Read the model definition and answer for the solid it produces. Units are mm, in the model's axes. A direction names the side the tool comes from. Coordinates: 2 decimals unless noted, no trailing zeros. Order: outer loops, then holes, each group sorted by start corner. A loop starts at its lowest first (then second) coordinate and runs counter-clockwise, first axis right, second up.
```python
from build123d import *

# Parameters (mm, degrees)
SKETCH1_R                = 10.975
SKETCH1_R_2              = 1.7
BOSS_EXTRUDE1_DEPTH      = 3.6
SKETCH2_R                = 5.125
BOSS_EXTRUDE2_DEPTH      = 13.7
BOSS_EXTRUDE3_DEPTH      = 13.7
BOSS_EXTRUDE3_DEPTH_BACK = 1.3
SKETCH2_2_R              = 5.125
CUT_EXTRUDE1_DEPTH       = 21.702445508
CUT_EXTRUDE1_DEPTH_BACK  = 21.702445508
SKETCH3_R                = 3.325
FILLET1_R                = 0.2
CHAMFER1_SIZE            = 0.2


with BuildPart() as part:
    # Sketch1 → Boss-Extrude1 (new body)
    with BuildSketch(Plane(origin=(0, 0, 0), x_dir=(0, 0, -1), z_dir=(1, 0, 0))):
        Circle(SKETCH1_R)
        with Locations((0, 7.775)):
            Circle(SKETCH1_R_2, mode=Mode.SUBTRACT)
        with Locations((7.775, 0)):
            Circle(SKETCH1_R_2, mode=Mode.SUBTRACT)
        with Locations((0, -7.775)):
            Circle(SKETCH1_R_2, mode=Mode.SUBTRACT)
        with Locations((-7.775, 0)):
            Circle(SKETCH1_R_2, mode=Mode.SUBTRACT)
    extrude(amount=BOSS_EXTRUDE1_DEPTH)

    # Sketch2 → Boss-Extrude2 (add)
    with BuildSketch(Plane(origin=(0, 0, 0), x_dir=(0, 0, -1), z_dir=(1, 0, 0))):
        with Locations(Location((0, 0, 0), (0, 0, 180))):
            Circle(SKETCH2_R)
    extrude(amount=BOSS_EXTRUDE2_DEPTH)

    # Sketch2_2 → Boss-Extrude3 (add, two sides: drawn at the far end of the back side and taken through both)
    with BuildSketch(Plane(origin=(0, 0, 0), x_dir=(0, 0, -1), z_dir=(1, 0, 0)).offset(-BOSS_EXTRUDE3_DEPTH_BACK)):
        with Locations(Location((0, 0, 0), (0, 0, 180))):
            Circle(SKETCH2_2_R)
    extrude(amount=BOSS_EXTRUDE3_DEPTH + BOSS_EXTRUDE3_DEPTH_BACK)

    # Sketch3 → Cut-Extrude1 (cut, two sides: drawn at the far end of the back side and taken through both)
    with BuildSketch(Plane(origin=(0, 0, 0), x_dir=(0, 0, -1), z_dir=(1, 0, 0)).offset(-CUT_EXTRUDE1_DEPTH_BACK)):
        Circle(SKETCH3_R)
    extrude(amount=CUT_EXTRUDE1_DEPTH + CUT_EXTRUDE1_DEPTH_BACK, mode=Mode.SUBTRACT)

    # Fillet1
    fillet1_edges = [part.edges().sort_by_distance(p)[0] for p in [
        (3.6, 0, -5.125),
    ]]
    fillet(fillet1_edges, radius=FILLET1_R)

    # Chamfer1
    chamfer1_edges = [part.edges().sort_by_distance(p)[0] for p in [
        (0, 0, 10.975),
        (13.7, 0, -5.125),
        (3.6, 0, 10.975),
    ]]
    chamfer(chamfer1_edges, length=CHAMFER1_SIZE)


solid = part.part
```
1) Which of the six approach directions +Z, -Z, +X, -X, +Y, -Y give full straight-line access (tool end or side, diameter ignored) to faces 1 (the flat face through (0, 5, 2)), 2 (the cylindrical face through (8.582, 1.963, 4.734)), 3 (the cylindrical face through (6.09, -2.95, -1.53))?
A:
face 1: -X
face 2: +X
face 3: +X, -X
2) A cutting plane is placed at A-A, the plane z = 0. State how many separate pieces and enclosed holes the cut face has, and give its area (3 significant figures).
A:
separate pieces: 4
enclosed holes: 0
area: 71.5 mm2
3) A cutting plane is placed at C-C, the plane x = 5. Determine the outline of the cut face in (y, z) (3 decimals), and give its area (3 significant figures).
A:
outline: circle Ø10.25 at (0, 0); hole circle Ø6.65 at (0, 0)
area: 47.8 mm2
4) Determine the mould class of faces 4 (the cylindrical face through (1.775, 6.115, 0.369)), 5 (the flat face through (-1.3, 3.3, 1.1)), 6 (the cylindrical face through (-0.659, 1.963, 4.734)) for opening direction Z: pulls with the +Z half, pulls with the -Z half, needs draft (parallel to the pull), parting line crosses it, or undercut.
A:
face 4: undercut
face 5: needs draft
face 6: parting line crosses it
5) Straight lines are drawn through the part: line 1 (X direction, y = -4.75, z = -5.25); line 2 (Y direction, x = 5.5, z = 0) (3 decimals); line 3 (Z direction, x = 9, y = 2.25). For each, find the intervals that lie inside material, in ascending order.
A:
line 1: x = 0 to 3.6
line 2: y = -5.125 to -3.325, 3.325 to 5.125
line 3: z = -4.6 to -2.45, 2.45 to 4.6
6) Flat-ended cylindrical pins translate along their axes: pin 1 Ø1.5 at (x, y) = (2, 1.5) entering from +Z; pin 2 Ø1.5 at (x, z) = (5.5, -5) entering from -Y; pin 3 Ø5 at (x, z) = (9.5, 2.5) entering from -Y (3 decimals). Find the tip coordinate at first contact, or state that the pin passes through.
A:
pin 1: stops at z = 10.95
pin 2: stops at y = -2.86
pin 3: stops at y = -5.125
